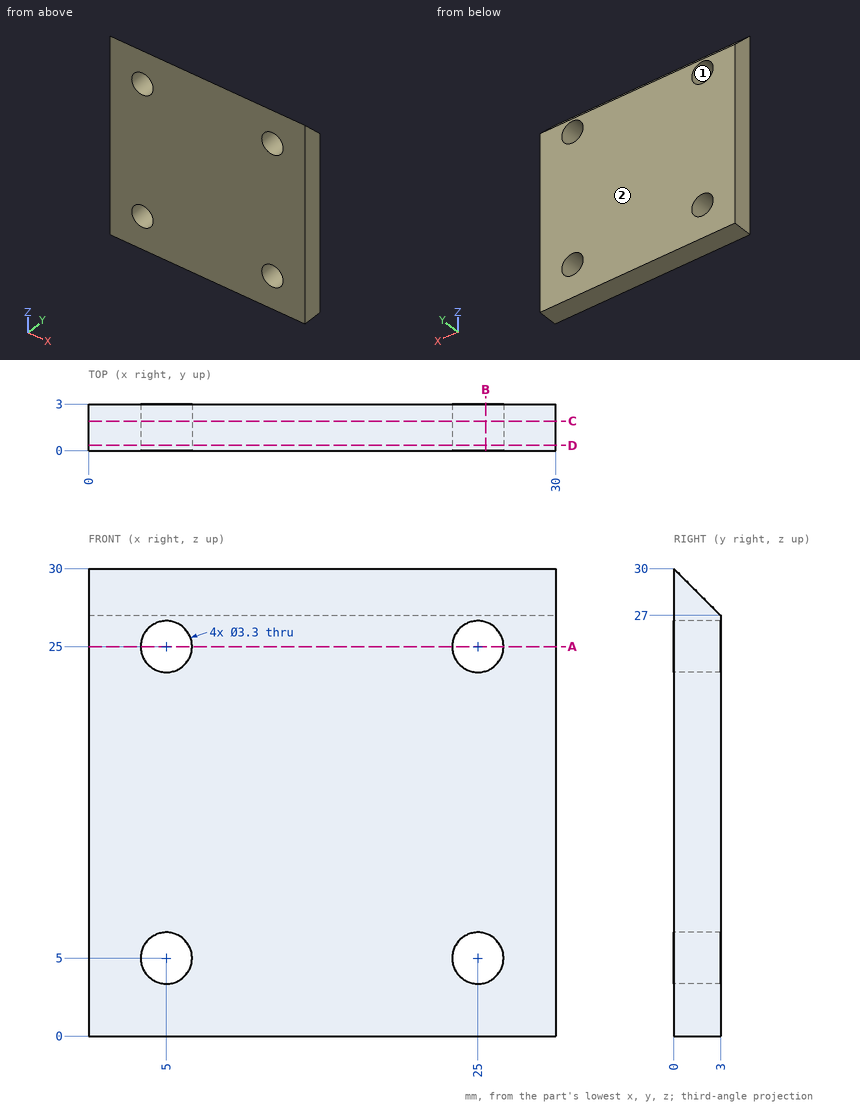
Part print with two shaded views. Sizes in mm from the minimum x, y, z corner. Round coordinates to 2 decimals unless told otherwise and drop trailing zeros. Write each loop counter-clockwise with the first axis right and the second up, starting at its lowest first coordinate (ties: lowest second). Pieces come first, ordered by that corner, then holes. Notation, with made-up numbers: (26, 56) -> (63, 56) arc R19 ccw to (63, 84) -> close; hole circle Ø4 at (22, 17.5). An arc over 180 degrees is marked (long way). Put each result on its own line as item: value.
Item 1: Slice it at D-D, the plane y = 0.35. Give the cut face in (x, z), plus the area to 3 significant figures.
Here are the results:
outline: (0, 0) -> (30, 0) -> (30, 29.65) -> (0, 29.65) -> close; hole circle Ø3.3 at (5, 5); hole circle Ø3.3 at (5, 25); hole circle Ø3.3 at (25, 5); hole circle Ø3.3 at (25, 25)
area: 855 mm^2
Item 2: Slice it at A-A, the plane z = 25. Give the cut face in (x, y), plus the area to 3 significant figures.
Here are the results:
outline: (0, 0) -> (3.35, 0) -> (3.35, 3) -> (0, 3) -> close; (6.65, 0) -> (23.35, 0) -> (23.35, 3) -> (6.65, 3) -> close; (26.65, 0) -> (30, 0) -> (30, 3) -> (26.65, 3) -> close
area: 70.2 mm^2
Item 3: Slice it at C-C, the plane y = 1.9. Give the cut face in (x, z).
Here are the results:
outline: (0, 0) -> (30, 0) -> (30, 28.1) -> (0, 28.1) -> close; hole circle Ø3.3 at (5, 5); hole circle Ø3.3 at (5, 25); hole circle Ø3.3 at (25, 5); hole circle Ø3.3 at (25, 25)
Item 4: Two-plate mould, pull along X, no slides. Class the marked faces 1 and 2: pulls with the +X half, pulls with the -X half, needs draft (parallel to the pull), parting line crosses it, or undercut.
Here are the results:
face 1: undercut
face 2: needs draft
Item 5: Slice it at B-B, the plane x = 25.5. Count the separate pieces of the cut face and the enclosed holes in it, plus the area to 3 significant figures.
Here are the results:
separate pieces: 3
enclosed holes: 0
area: 66.6 mm^2
Item 6: Wall check: probe 1 along X at (y, z) = (1.55, 25); probe 2 along Z at (x, y) = (6.5, 2.1); probe 3 along Z at (x, y) = (25, 2.1). Give the ranges that are in metal, low to high. Write a range as from..to.
Here are the results:
probe 1: x = 0..3.35, 6.65..23.35, 26.65..30
probe 2: z = 0..4.31, 5.69..24.31, 25.69..27.9
probe 3: z = 0..3.35, 6.65..23.35, 26.65..27.9
Item 7: Flat gauge pin, fed straight in: P1, Ø1, axis at x = 13.5, y = 1.5, coming from the +Z side. Where does the tip first touch, or does it go through?
Here are the results:
P1: stops at z = 29
